from build123d import *

# Parameters (mm, degrees)
SKETCH1_R           = 50
BOSS_EXTRUDE1_DEPTH = 25
CUT_EXTRUDE1_DEPTH  = 18.25


with BuildPart() as part:
    # Sketch1 → Boss-Extrude1 (new body)
    with BuildSketch(Plane(origin=(0, 0, 0), x_dir=(1, 0, 0), z_dir=(0, 1, 0))):
        with Locations(Location((0, 0, 0), (0, 0, 270))):
            Circle(SKETCH1_R)
    extrude(amount=-BOSS_EXTRUDE1_DEPTH)

    # Sketch2 → Cut-Extrude1 (cut)
    with BuildSketch(Plane(origin=(0, 0, 0), x_dir=(1, 0, 0), z_dir=(0, 1, 0))):
        with BuildLine():
            Line((-20.85, 39.78798688), (-17.461642921, 33.321996136))
            ThreePointArc((-17.461642921, 33.321996136), (-34.039720295, 16.017547946), (-36.805386336, -7.786394331))
            Line((-36.805386336, -7.786394331), (-31.645347938, -7.786394331))
            ThreePointArc((-31.645347938, -7.786394331), (-28.461211468, -15.874993686), (-23.252089779, -22.834103961))
            Line((-23.252089779, -22.834103961), (-32.05, -31.473860583))
            ThreePointArc((-32.05, -31.473860583), (0, -44.92), (32.05, -31.473860583))
            Line((32.05, -31.473860583), (26.841518255, -26.359007906))
            ThreePointArc((26.841518255, -26.359007906), (37.154813328, -5.897817101), (33.684688853, 16.751302542))
            Line((33.684688853, 16.751302542), (27.954424443, 16.751302542))
            ThreePointArc((27.954424443, 16.751302542), (25.023160627, 20.878156409), (21.488186441, 24.501302542))
            ThreePointArc((21.488186441, 24.501302542), (18.436983495, 26.872544025), (15.126554505, 28.865954542))
            Line((15.126554505, 28.865954542), (20.85, 39.78798688))
            ThreePointArc((20.85, 39.78798688), (0, 44.92), (-20.85, 39.78798688))
        make_face()
    extrude(amount=-CUT_EXTRUDE1_DEPTH, mode=Mode.SUBTRACT)


solid = part.part
Here's how the part is built. I have some questions about the finished solid (model axes, mm). A direction names the side the tool comes from. Round coordinates to 2 decimals unless told otherwise and drop trailing zeros. Order: outer loops, then holes, each group sorted by start corner. A loop starts at its lowest first (then second) coordinate and runs counter-clockwise, first axis right, second up. Notation, with made-up numbers: M 85,60 L 124,60 A19 ccw 124,68 Z; hole C 74.25,-13.75 d3. An arc over 180 degrees is marked long. Return JSON: item names as keys, results as strings. Group by question number.
1. If we section it at A-A on y = -17: List the corners of the cut face in (x, z) for me.
2. If we section it at D-D on y = -23: List the corners of the cut face in (x, z) for me, then the cut area to 3 significant figures.
3. On a 3-axis mill with a long thin cutter (end or side, diameter ignored), from which of +Z, -Z, +X, -X, +Y, -Y can I reach the whole of each face in a straight line? I mean faces 1 (the face through (1, -25, -1)), 2 (the face through (31, -9, -16.751)). Say none if no direction works.
4. If we section it at C-C on z = 0: List the corners of the cut face in (x, y) for me, then the cut area to 3 significant figures.
5. I'm going to push flat-ended pins straight in: pin 1 Ø1 at (x, y) = (-6.5, -14) entering from +Z; pin 2 Ø2 at (y, z) = (-14.5, 39.5) entering from -X; pin 3 Ø4.5 at (x, y) = (29.5, -9.5) entering from +Z. Where does each tip first touch, or does it pass through?
6. Please list where these lines run through material, in increasing order: probe 1 along X at (y, z) = (-11.25, 21); probe 2 along X at (y, z) = (-14.5, -14); probe 3 along Z at (x, y) = (-25, -11).
7. If we mould it in two halves opening along Z, with no side actions, what happens to faces 3 (the face through (15.02, -12.32, 47.69)), 4 (the face through (22, 0, -26)), 5 (the face through (29.48, -9, 28.95)), 6 (the face through (0.3, -9, -44.92))? For each: pulls with the +Z half, pulls with the -Z half, needs draft (parallel to the pull), parting line crosses it, or undercut.
8. If we section it at B-B on x = 0: List the corners of the cut face in (y, z) for me.
Reply:
{
 "1": {"outline": "C 0,0 d100; hole M -36.81,7.79 A37.62 ccw -17.46,-33.32 L -20.85,-39.79 A44.92 ccw 20.85,-39.79 L 15.13,-28.87 A32.59 ccw 27.95,-16.75 L 33.68,-16.75 A37.62 ccw 26.84,26.36 L 32.05,31.47 A44.92 ccw -32.05,31.47 L -23.25,22.83 A32.59 ccw -31.65,7.79 Z"},
 "2": {"outline": "C 0,0 d100", "area": "7,850 mm^2"},
 "3": {"face 1": "+Z, -Z, +X, -X, -Y", "face 2": "+Y"},
 "4": {"outline": "M -50,-25 L 50,-25 L 50,0 L 37.62,0 L 37.62,-18.25 L -37.62,-18.25 L -37.62,0 L -50,0 Z", "area": "1,130 mm^2"},
 "5": {"pin 1": "z = 49.64", "pin 2": "x = -31.9", "pin 3": "z = 41.92"},
 "6": {"probe 1": "-45.38 to -24.92, 31.21 to 45.38", "probe 2": "-48 to -34.92, 34.92 to 48", "probe 3": "-43.3 to -28.11, 20.91 to 24.55, 37.32 to 43.3"},
 "7": {"face 3": "parting line crosses it", "face 4": "needs draft", "face 5": "undercut", "face 6": "undercut"},
 "8": {"outline": "M -25,-50 L 0,-50 L 0,-44.92 L -18.25,-44.92 L -18.25,44.92 L 0,44.92 L 0,50 L -25,50 Z"}
}
